Source: CAD feature listing. Evaluate the final solid. Frame: model axes, mm. A direction names the side the tool comes from. Give positions to 0.01 mm unless a question says otherwise; leave off trailing zeros. Loops run counter-clockwise (first coordinate to the right, second up) from the corner with the lowest first, then second, coordinate; pieces in that order, holes last. Notation, with made-up numbers: (5, 28) - (11, 28) arc R12 cw to (11, 41) - close; hole circle Ø2 at (-25, -39.5). An arc over 180 degrees is marked (long way). Put each result on its own line as item: value.
```python
from build123d import *

# Parameters (mm, degrees)
F1_DEPTH    = 5
F2_T1_DEPTH = 55
F2_T3_DEPTH = 54.7482455069
F2_T5_DEPTH = 54.435996907


# Not quite as in the source:
# - a fillet or chamfer that OpenCascade refuses, or shapes differently, is made with other operations: its cross-section is extruded or revolved along the edge and cut away or added


with BuildPart() as f1:
    # F0 (on Front) → F1 (new body)
    with BuildSketch(Plane.XZ):
        Polygon((2.5022388734, -13.5), (11.5, -13.5), (11.5, 13.5), (-11.5, 13.5), (-11.5, -13.5), (-2.9977611266, -13.5), (-2.9977611266, 0), (2.5022388734, 0), align=None)
    extrude(amount=F1_DEPTH)

    # F2: fillet of radius 10 on 4 edges, made by hand

    # F2_s2 → F2_t1 (cut)
    with BuildSketch(Plane.XZ.offset(-25)):
        with BuildLine():
            ThreePointArc((-1.5, 13.5), (-8.5710678119, 10.5710678119), (-11.5, 3.5))
            Line((-11.5, 3.5), (-11.5, 13.5))
            Line((-11.5, 13.5), (-1.5, 13.5))
        make_face()
        with BuildLine():
            ThreePointArc((11.5, 3.5), (8.5710678119, 10.5710678119), (1.5, 13.5))
            Line((1.5, 13.5), (11.5, 13.5))
            Line((11.5, 13.5), (11.5, 3.5))
        make_face()
    extrude(amount=F2_T1_DEPTH, mode=Mode.SUBTRACT)

    # F2_s4 → F2_t3 (cut)
    with BuildSketch(Plane.XZ.offset(-24.8741227535)):
        with BuildLine():
            ThreePointArc((2.5022388734, -13.5), (8.9169531728, -10.2577204004), (11.5, -3.5503508986))
            Line((11.5, -3.5503508986), (11.5, -13.5))
            Line((11.5, -13.5), (2.5022388734, -13.5))
        make_face()
    extrude(amount=F2_T3_DEPTH, mode=Mode.SUBTRACT)

    # F2_s6 → F2_t5 (cut)
    with BuildSketch(Plane.XZ.offset(-24.7179984535)):
        with BuildLine():
            ThreePointArc((-11.5, -3.6128006186), (-9.0821372734, -10.132861536), (-2.9977611266, -13.5))
            Line((-2.9977611266, -13.5), (-11.5, -13.5))
            Line((-11.5, -13.5), (-11.5, -3.6128006186))
        make_face()
    extrude(amount=F2_T5_DEPTH, mode=Mode.SUBTRACT)


solid = f1.part
```
1) Section query C-C, the plane z = -9.75. Output: boundary loops of the cut face in (x, y), plus the area to 3 significant figures.
Check result:
outline: (-9.4, -5) - (-3, -5) - (-3, 0) - (-9.4, 0) - close; (2.5, -5) - (9.35, -5) - (9.35, 0) - (2.5, 0) - close
area: 66.2 mm²
2) Access query for faces 5 (the flat face through (0, -2, 13.5)), 6 (the flat face through (0, -2, 0)). Directions: +Z, -Z, +X, -X, +Y, -Y. A direction counts if a zero-diameter tool reaches every point of the face in a straight line with its end or side. Return the directions, or none.
Check result:
face 5: +Z, +X, -X, +Y, -Y
face 6: -Z, +Y, -Y
3) Mould query, pull axis X, two halves, no side actions, for faces 1 (the flat face through (-2.998, -2, -7)), 2 (the cylindrical face through (8.85, -2.46, -10.33)), 3 (the flat face through (2.502, -2, -7)), 4 (the cylindrical face through (-9.147, -2.465, -10.057)). Classes: pulls with the +X half, pulls with the -X half, needs draft (parallel to the pull), parting line crosses it, or undercut.
Check result:
face 1: undercut
face 2: pulls with the +X half
face 3: undercut
face 4: pulls with the -X half
4) Section query A-A, the plane y = -1.2. Output: boundary loops of the cut face in (x, z), plus the area to 3 significant figures.
Check result:
outline: (-11.5, -3.61) arc R10 ccw to (-3, -13.5) - (-3, 0) - (2.5, 0) - (2.5, -13.5) arc R10 ccw to (11.5, -3.55) - (11.5, 3.5) arc R10 ccw to (1.5, 13.5) - (-1.5, 13.5) arc R10 ccw to (-11.5, 3.5) - close
area: 462 mm²
5) Section query B-B, the plane z = -7. Output: boundary loops of the cut face in (x, y).
Check result:
outline: (-10.91, -5) - (-3, -5) - (-3, 0) - (-10.91, 0) - close; (2.5, -5) - (10.89, -5) - (10.89, 0) - (2.5, 0) - close
6) Pin query (flat end, axial travel): P1, Ø1.5, axis at x = 8.5, y = -3.5, coming from the +Z side; P2, Ø2, axis at y = -2.5, z = -8.5, coming from the +X side; P3, Ø2.5, axis at x = -1, y = -2, coming from the -Z side. Return the tip coordinate at first contact, or that it passes through.
Check result:
P1: z = 11.31
P2: x = 10.69
P3: z = 0
7) Material intervals for line 1 along X through (y, z) = (-2.05, -3.25); line 2 along X through (y, z) = (-2.5, 3.75); line 3 along X through (y, z) = (-3.3, -11), sorted ascending. Write a range as [from, to].
Check result:
line 1: [-11.5, -3], [2.5, 11.5]
line 2: [-11.5, 11.5]
line 3: [-8.24, -3], [2.5, 8.17]
8) Section query D-D, the plane x = -0.5. Output: boundary loops of the cut face in (y, z).
Check result:
outline: (-5, 0) - (0, 0) - (0, 13.5) - (-5, 13.5) - close
